Geometry: final body of the model. Coordinates: model frame, mm. A direction names the side the tool comes from. Coordinates: 2 decimals unless noted, no trailing zeros. Order: outer loops, then holes, each group sorted by start corner. A loop starts at its lowest first (then second) coordinate and runs counter-clockwise, first axis right, second up. Notation, with made-up numbers: (77.25, -24.5) - (115.25, -24.5) arc R22 cw to (115.25, 6.5) - close; hole circle Ø2 at (88.5, 50). An arc over 180 degrees is marked (long way). Use one line per item in the form item = value. Start each with the question number.
```python
from build123d import *

# Parameters (mm, degrees)
ESBO_O1_W                     = 130
ESBO_O1_H                     = 32
RESSALTO_EXTRUS_O1_DEPTH      = 10
RESSALTO_EXTRUS_O1_DEPTH_BACK = 10
ESBO_O2_W                     = 90
ESBO_O2_H                     = 20
CORTE_EXTRUS_O1_DEPTH         = 21
FILETE1_R                     = 10
ESBO_O4_R                     = 4
CORTE_EXTRUS_O2_DEPTH         = 29.5
ESBO_O5_R                     = 2.25
CORTE_EXTRUS_O3_DEPTH         = 33


with BuildPart() as part:
    # Esbo_o1 → Ressalto-extrus_o1 (new body, two sides)
    with BuildSketch(Plane.XY) as ressalto_extrus_o1_sk:
        Rectangle(ESBO_O1_W, ESBO_O1_H)
    extrude(amount=RESSALTO_EXTRUS_O1_DEPTH)
    extrude(ressalto_extrus_o1_sk.sketch, amount=-RESSALTO_EXTRUS_O1_DEPTH_BACK)

    # Esbo_o2 → Corte-extrus_o1 (cut, through all)
    with BuildSketch(Plane.XY.offset(10)):
        Polygon((35, 16), (55, 6.308022976), (65, -16), (65, 16), align=None)
        Polygon((-65, -16), (-65, 16), (-35, 16), (-55, 6.308022976), align=None)
        with Locations((0, -6)):
            Rectangle(ESBO_O2_W, ESBO_O2_H)
    extrude(amount=-CORTE_EXTRUS_O1_DEPTH, mode=Mode.SUBTRACT)

    # Filete1
    filete1_edges = [part.edges().sort_by_distance(p)[0] for p in [
        (-55, 6.308022976, 0),
        (-35, 16, 0),
        (45, 4, 0),
        (-45, 4, 0),
        (35, 16, 0),
        (55, 6.308022976, 0),
    ]]
    fillet(filete1_edges, radius=FILETE1_R)

    # Esbo_o4 → Corte-extrus_o2 (cut)
    with BuildSketch(Plane(origin=(0, 16, 0), x_dir=(1, 0, 0), z_dir=(0, 1, 0))):
        with Locations((-55, 0)):
            Circle(ESBO_O4_R)
        with Locations((55, 0)):
            Circle(ESBO_O4_R)
    extrude(amount=-CORTE_EXTRUS_O2_DEPTH, mode=Mode.SUBTRACT)

    # Esbo_o5 → Corte-extrus_o3 (cut, through all)
    with BuildSketch(Plane(origin=(0, 16, 0), x_dir=(1, 0, 0), z_dir=(0, 1, 0))):
        with Locations((-55, 0)):
            Circle(ESBO_O5_R)
        with Locations((55, 0)):
            Circle(ESBO_O5_R)
    extrude(amount=-CORTE_EXTRUS_O3_DEPTH, mode=Mode.SUBTRACT)


solid = part.part
```
(1) Contact query for flat-ended pins moving along their axis: pin 1 Ø10 at (x, z) = (40, 7.5) entering from +Y; pin 2 Ø7 at (x, z) = (-55, 0) entering from +Y; pin 3 Ø10 at (y, z) = (12, -3) entering from -X; pin 4 Ø2.5 at (x, z) = (55, 0) entering from -Y. Output: stop coordinate, or through.
(2) Set-up query: faces 3 (the cylindrical face through (34.911, 15.754, -0.14)), 4 (the flat face through (45, -11, 0)), 5 (the flat face through (57, -13.5, 2)). Return all of +Z, -Z, +X, -X, +Y, -Y with unobstructed straight access to the full face (end or side cutting, diameter ignored); none if empty.
(3) Material intervals for L1, parallel to X at y = -15.25, z = 0; L2, parallel to Z at x = -55, y = -14; L3, parallel to X at y = -8, z = 0, sorted ascending. Write a range as from..to.
(4) Cut plane B-B on z = -7. Return the cut outline in (x, y), plus the area to 3 significant figures.
(5) Cut plane A-A on y = -10.5. Return the cut outline in (x, z).
(6) Cut plane D-D on z = 0. Return the cut outline in (x, y).
(7) Draft query along Z for faces 1 (the cylindrical face through (-51.185, -4.891, -1.201)), 2 (the flat face through (-60.685, -6.374, 0.14)). Return one class per face: released by +Z, released by -Z, zero draft, split by the parting line, or undercut.
(8) Cut plane C-C on x = -55. Return the cut outline in (y, z).
Check sheet entries:
q1.pin_1 = 15.73
q1.pin_2 = -13.5
q1.pin_3 = -53.18
q1.pin_4 = through
q2.face_3 = +Z, -Z, +X, +Y
q2.face_4 = +Z, -Z, -Y
q2.face_5 = +Y
q3.L1 = -64.66..-57.25, -52.75..-45, 45..52.75, 57.25..64.66
q3.L2 = -10..-2.25, 2.25..10
q3.L3 = -61.41..-59, -51..-45, 45..51, 59..61.41
q4.outline = (-65, -16) - (-45, -16) - (-45, -6) arc R10 cw to (-35, 4) - (35, 4) arc R10 cw to (45, -6) - (45, -16) - (65, -16) - (56.49, 2.99) arc R10 ccw to (51.72, 7.9) - (37.07, 15) arc R10 ccw to (32.7, 16) - (-32.7, 16) arc R10 ccw to (-37.07, 15) - (-51.72, 7.9) arc R10 ccw to (-56.49, 2.99) - close
q4.area = 1,790 mm^2
q5.outline = (-62.53, -10) - (-45, -10) - (-45, 10) - (-62.53, 10) - close; (45, -10) - (62.53, -10) - (62.53, 10) - (45, 10) - close; hole circle Ø8 at (-55, 0); hole circle Ø8 at (55, 0)
q6.outline = (-65, -16) - (-57.25, -16) - (-57.25, -13.5) - (-59, -13.5) - (-59, -2.62) - close; (-52.75, -16) - (-45, -16) - (-45, -6) arc R10 cw to (-35, 4) - (35, 4) arc R10 cw to (45, -6) - (45, -16) - (52.75, -16) - (52.75, -13.5) - (51, -13.5) - (51, 8.25) - (37.07, 15) arc R10 ccw to (32.7, 16) - (-32.7, 16) arc R10 ccw to (-37.07, 15) - (-51, 8.25) - (-51, -13.5) - (-52.75, -13.5) - close; (57.25, -16) - (65, -16) - (59, -2.62) - (59, -13.5) - (57.25, -13.5) - close
q7.face_1 = undercut
q7.face_2 = zero draft
q8.outline = (-16, -10) - (5.35, -10) - (5.35, -4) - (-13.5, -4) - (-13.5, -2.25) - (-16, -2.25) - close; (-16, 2.25) - (-13.5, 2.25) - (-13.5, 4) - (5.35, 4) - (5.35, 10) - (-16, 10) - close
